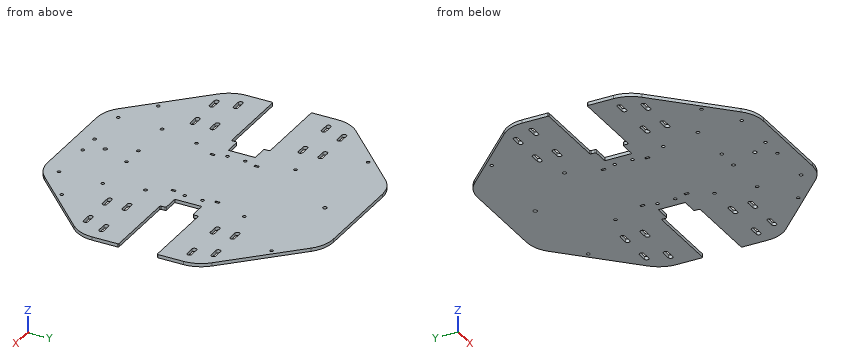
from build123d import *

# Parameters (mm, degrees)
SKETCH1_R           = 1.85
SKETCH1_R_2         = 1.5
BOSS_EXTRUDE1_DEPTH = 3
SKETCH2_R           = 1.5
SKETCH2_W           = 2
SKETCH2_H           = 4
CUT_EXTRUDE1_DEPTH  = 10
FILLET1_R           = 1
FILLET2_R           = 1
SKETCH3_R           = 1.5
CUT_EXTRUDE2_DEPTH  = 10


with BuildPart() as part:
    # Sketch1 → Boss-Extrude1 (new body)
    with BuildSketch(Plane.XY):
        with BuildLine():
            Line((130, 17.5), (130, 41.421356237))
            ThreePointArc((130, 41.421356237), (127.716385975, 52.901859208), (121.213203436, 62.634559673))
            Line((121.213203436, 62.634559673), (62.634559673, 121.213203436))
            ThreePointArc((62.634559673, 121.213203436), (52.901859208, 127.716385975), (41.421356237, 130))
            Line((41.421356237, 130), (-41.421356237, 130))
            ThreePointArc((-41.421356237, 130), (-52.901859208, 127.716385975), (-62.634559673, 121.213203436))
            Line((-62.634559673, 121.213203436), (-121.213203436, 62.634559673))
            ThreePointArc((-121.213203436, 62.634559673), (-127.716385975, 52.901859208), (-130, 41.421356237))
            Line((-130, 41.421356237), (-130, 17.5))
            Line((-130, 17.5), (-60, 17.5))
            Line((-60, 17.5), (-60, 12.25))
            Line((-60, 12.25), (-45, 12.25))
            Line((-45, 12.25), (-45, -12.25))
            Line((-45, -12.25), (-60, -12.25))
            Line((-60, -12.25), (-60, -17.5))
            Line((-60, -17.5), (-130, -17.5))
            Line((-130, -17.5), (-130, -41.421356237))
            ThreePointArc((-130, -41.421356237), (-127.716385975, -52.901859208), (-121.213203436, -62.634559673))
            Line((-121.213203436, -62.634559673), (-62.634559673, -121.213203436))
            ThreePointArc((-62.634559673, -121.213203436), (-52.901859208, -127.716385975), (-41.421356237, -130))
            Line((-41.421356237, -130), (41.421356237, -130))
            ThreePointArc((41.421356237, -130), (52.901859208, -127.716385975), (62.634559673, -121.213203436))
            Line((62.634559673, -121.213203436), (121.213203436, -62.634559673))
            ThreePointArc((121.213203436, -62.634559673), (127.716385975, -52.901859208), (130, -41.421356237))
            Line((130, -41.421356237), (130, -17.5))
            Line((130, -17.5), (60, -17.5))
            Line((60, -17.5), (60, -12.25))
            Line((60, -12.25), (45, -12.25))
            Line((45, -12.25), (45, 12.25))
            Line((45, 12.25), (60, 12.25))
            Line((60, 12.25), (60, 17.5))
            Line((60, 17.5), (130, 17.5))
        make_face()
        with Locations((0, 100)):
            Circle(SKETCH1_R, mode=Mode.SUBTRACT)
        with Locations(Location((0, -100, 0), (0, 0, 180))):
            Circle(SKETCH1_R, mode=Mode.SUBTRACT)
        with Locations((36, 8.1)):
            Circle(SKETCH1_R_2, mode=Mode.SUBTRACT)
        with Locations(Location((36, -8.1, 0), (0, 0, 180))):
            Circle(SKETCH1_R_2, mode=Mode.SUBTRACT)
        with Locations((-36, -8.1)):
            Circle(SKETCH1_R_2, mode=Mode.SUBTRACT)
        with Locations(Location((-36, 8.1, 0), (0, 0, 180))):
            Circle(SKETCH1_R_2, mode=Mode.SUBTRACT)
        with BuildLine():
            Line((69.925, 42.0875), (78.075, 42.0875))
            ThreePointArc((78.075, 42.0875), (80.1125, 40.05), (78.075, 38.0125))
            Line((78.075, 38.0125), (69.925, 38.0125))
            ThreePointArc((69.925, 38.0125), (67.8875, 40.05), (69.925, 42.0875))
        make_face(mode=Mode.SUBTRACT)
        with BuildLine():
            Line((69.925, 60.1375), (78.075, 60.1375))
            ThreePointArc((78.075, 60.1375), (80.1125, 58.1), (78.075, 56.0625))
            Line((78.075, 56.0625), (69.925, 56.0625))
            ThreePointArc((69.925, 56.0625), (67.8875, 58.1), (69.925, 60.1375))
        make_face(mode=Mode.SUBTRACT)
        with BuildLine():
            Line((101.925, 60.1375), (110.075, 60.1375))
            ThreePointArc((110.075, 60.1375), (112.1125, 58.1), (110.075, 56.0625))
            Line((110.075, 56.0625), (101.925, 56.0625))
            ThreePointArc((101.925, 56.0625), (99.8875, 58.1), (101.925, 60.1375))
        make_face(mode=Mode.SUBTRACT)
        with BuildLine():
            Line((108.925, 42.0875), (117.075, 42.0875))
            ThreePointArc((117.075, 42.0875), (119.1125, 40.05), (117.075, 38.0125))
            Line((117.075, 38.0125), (108.925, 38.0125))
            ThreePointArc((108.925, 38.0125), (106.8875, 40.05), (108.925, 42.0875))
        make_face(mode=Mode.SUBTRACT)
        with BuildLine():
            Line((-69.925, 60.1375), (-78.075, 60.1375))
            ThreePointArc((-78.075, 60.1375), (-80.1125, 58.1), (-78.075, 56.0625))
            Line((-78.075, 56.0625), (-69.925, 56.0625))
            ThreePointArc((-69.925, 56.0625), (-67.8875, 58.1), (-69.925, 60.1375))
        make_face(mode=Mode.SUBTRACT)
        with BuildLine():
            Line((-101.925, 60.1375), (-110.075, 60.1375))
            ThreePointArc((-110.075, 60.1375), (-112.1125, 58.1), (-110.075, 56.0625))
            Line((-110.075, 56.0625), (-101.925, 56.0625))
            ThreePointArc((-101.925, 56.0625), (-99.8875, 58.1), (-101.925, 60.1375))
        make_face(mode=Mode.SUBTRACT)
        with BuildLine():
            Line((-108.925, 42.0875), (-117.075, 42.0875))
            ThreePointArc((-117.075, 42.0875), (-119.1125, 40.05), (-117.075, 38.0125))
            Line((-117.075, 38.0125), (-108.925, 38.0125))
            ThreePointArc((-108.925, 38.0125), (-106.8875, 40.05), (-108.925, 42.0875))
        make_face(mode=Mode.SUBTRACT)
        with BuildLine():
            Line((-69.925, 42.0875), (-78.075, 42.0875))
            ThreePointArc((-78.075, 42.0875), (-80.1125, 40.05), (-78.075, 38.0125))
            Line((-78.075, 38.0125), (-69.925, 38.0125))
            ThreePointArc((-69.925, 38.0125), (-67.8875, 40.05), (-69.925, 42.0875))
        make_face(mode=Mode.SUBTRACT)
        with BuildLine():
            Line((101.925, -60.1375), (110.075, -60.1375))
            ThreePointArc((110.075, -60.1375), (112.1125, -58.1), (110.075, -56.0625))
            Line((110.075, -56.0625), (101.925, -56.0625))
            ThreePointArc((101.925, -56.0625), (99.8875, -58.1), (101.925, -60.1375))
        make_face(mode=Mode.SUBTRACT)
        with BuildLine():
            Line((69.925, -60.1375), (78.075, -60.1375))
            ThreePointArc((78.075, -60.1375), (80.1125, -58.1), (78.075, -56.0625))
            Line((78.075, -56.0625), (69.925, -56.0625))
            ThreePointArc((69.925, -56.0625), (67.8875, -58.1), (69.925, -60.1375))
        make_face(mode=Mode.SUBTRACT)
        with BuildLine():
            Line((69.925, -42.0875), (78.075, -42.0875))
            ThreePointArc((78.075, -42.0875), (80.1125, -40.05), (78.075, -38.0125))
            Line((78.075, -38.0125), (69.925, -38.0125))
            ThreePointArc((69.925, -38.0125), (67.8875, -40.05), (69.925, -42.0875))
        make_face(mode=Mode.SUBTRACT)
        with BuildLine():
            Line((108.925, -42.0875), (117.075, -42.0875))
            ThreePointArc((117.075, -42.0875), (119.1125, -40.05), (117.075, -38.0125))
            Line((117.075, -38.0125), (108.925, -38.0125))
            ThreePointArc((108.925, -38.0125), (106.8875, -40.05), (108.925, -42.0875))
        make_face(mode=Mode.SUBTRACT)
        with BuildLine():
            Line((-101.925, -60.1375), (-110.075, -60.1375))
            ThreePointArc((-110.075, -60.1375), (-112.1125, -58.1), (-110.075, -56.0625))
            Line((-110.075, -56.0625), (-101.925, -56.0625))
            ThreePointArc((-101.925, -56.0625), (-99.8875, -58.1), (-101.925, -60.1375))
        make_face(mode=Mode.SUBTRACT)
        with BuildLine():
            Line((-69.925, -60.1375), (-78.075, -60.1375))
            ThreePointArc((-78.075, -60.1375), (-80.1125, -58.1), (-78.075, -56.0625))
            Line((-78.075, -56.0625), (-69.925, -56.0625))
            ThreePointArc((-69.925, -56.0625), (-67.8875, -58.1), (-69.925, -60.1375))
        make_face(mode=Mode.SUBTRACT)
        with BuildLine():
            Line((-69.925, -42.0875), (-78.075, -42.0875))
            ThreePointArc((-78.075, -42.0875), (-80.1125, -40.05), (-78.075, -38.0125))
            Line((-78.075, -38.0125), (-69.925, -38.0125))
            ThreePointArc((-69.925, -38.0125), (-67.8875, -40.05), (-69.925, -42.0875))
        make_face(mode=Mode.SUBTRACT)
        with BuildLine():
            Line((-108.925, -42.0875), (-117.075, -42.0875))
            ThreePointArc((-117.075, -42.0875), (-119.1125, -40.05), (-117.075, -38.0125))
            Line((-117.075, -38.0125), (-108.925, -38.0125))
            ThreePointArc((-108.925, -38.0125), (-106.8875, -40.05), (-108.925, -42.0875))
        make_face(mode=Mode.SUBTRACT)
    extrude(amount=BOSS_EXTRUDE1_DEPTH)

    # Sketch2 → Cut-Extrude1 (cut)
    with BuildSketch(Plane.XY.offset(3)):
        with Locations((-10, -75.1)):
            Circle(SKETCH2_R)
        with Locations((-49.9, -75.1)):
            Circle(SKETCH2_R)
        with Locations((-10, -115)):
            Circle(SKETCH2_R)
        with Locations((-49.9, -115)):
            Circle(SKETCH2_R)
        with Locations((10, -75.1)):
            Circle(SKETCH2_R)
        with Locations((49.9, -75.1)):
            Circle(SKETCH2_R)
        with Locations((49.9, -115)):
            Circle(SKETCH2_R)
        with Locations((10, -115)):
            Circle(SKETCH2_R)
        with Locations((33, -20)):
            Rectangle(SKETCH2_W, SKETCH2_H)
        with Locations((33, 20)):
            Rectangle(SKETCH2_W, SKETCH2_H)
        with Locations((-33, 20)):
            Rectangle(SKETCH2_W, SKETCH2_H)
        with Locations((-33, -20)):
            Rectangle(SKETCH2_W, SKETCH2_H)
    extrude(amount=-CUT_EXTRUDE1_DEPTH, mode=Mode.SUBTRACT)

    # Fillet1
    fillet1_edges = [part.edges().sort_by_distance(p)[0] for p in [
        (130, 17.5, 1.5),
        (60, 17.5, 1.5),
        (60, 12.25, 1.5),
        (60, -12.25, 1.5),
        (60, -17.5, 1.5),
        (130, -17.5, 1.5),
    ]]
    fillet(fillet1_edges, radius=FILLET1_R)

    # Fillet2
    fillet2_edges = [part.edges().sort_by_distance(p)[0] for p in [
        (-130, -17.5, 1.5),
        (-60, -17.5, 1.5),
        (-60, -12.25, 1.5),
        (-60, 12.25, 1.5),
        (-60, 17.5, 1.5),
        (-130, 17.5, 1.5),
    ]]
    fillet(fillet2_edges, radius=FILLET2_R)

    # Sketch3 → Cut-Extrude2 (cut)
    with BuildSketch(Plane.XY.offset(3)):
        with Locations((-43, 50)):
            Circle(SKETCH3_R)
        with Locations((-43, -40)):
            Circle(SKETCH3_R)
        with Locations((43, -40)):
            Circle(SKETCH3_R)
        with Locations((43, 50)):
            Circle(SKETCH3_R)
        with Locations((-81.317279836, 95.45941546)):
            Circle(SKETCH3_R)
        with Locations((81.317279836, 95.45941546)):
            Circle(SKETCH3_R)
        with Locations((81.317279836, -95.45941546)):
            Circle(SKETCH3_R)
        with Locations((-81.317279836, -95.45941546)):
            Circle(SKETCH3_R)
    extrude(amount=-CUT_EXTRUDE2_DEPTH, mode=Mode.SUBTRACT)


solid = part.part
Can you work these out from the model? Positions are in its coordinate system, mm. Give positions to 0.01 mm unless a question says otherwise; leave off trailing zeros. Loops run counter-clockwise (first coordinate to the right, second up) from the corner with the lowest first, then second, coordinate; pieces in that order, holes last. Notation, with made-up numbers: (26, -14.5) - (44, -14.5) arc R24 ccw to (44, -4.5) - close; hole circle Ø3 at (61, 1.5). An arc over 180 degrees is marked (long way). Answer as a JSON object with one key per item and string values.
Q1. Will these pins go through, and if not, where does the flat tip stop? P1, Ø0.9, axis at x = 108, z = 2, coming from the -Y side; P2, Ø1, axis at x = -46.5, z = 2.5, coming from the +Y side; P3, Ø1.5, axis at x = 105, z = 1.5, coming from the +Y side.
Geometry says:
{"P1": "y = -76.3", "P2": "y = 129.65", "P3": "y = 79.6"}
Q2. Imagine slicing it at C-C on y = 77.5. Write out the boundary of the cut face in (x, z), plus the area to 3 significant figures.
Geometry says:
{"outline": "(-106.35, 0) - (106.35, 0) - (106.35, 3) - (-106.35, 3) - close", "area": "638 mm²"}
Q3. If I drill on L1, parallel to X at y = -21, z = 2.6; L2, parallel to Y at x = 10, z = 1.3; L3, parallel to Y at x = 36, z = 0.7, over which ranges is the centre line in solid material (lowest first)?
Geometry says:
{"L1": "-130 to -34, -32 to 32, 34 to 130", "L2": "-130 to -116.5, -113.5 to -76.6, -73.6 to 130", "L3": "-130 to -9.6, -6.6 to 6.6, 9.6 to 130"}
Q4. Imagine slicing it at A-A on z = 1. Give the number of separate pieces and of enclosed holes in the cut face, plus the area to 3 significant figures.
Geometry says:
{"separate pieces": "1", "enclosed holes": "42", "area": "49,300 mm²"}
Q5. Imagine slicing it at B-B on y = -108.5. Write out the boundary of the cut face in (x, z), plus the area to 3 significant figures.
Geometry says:
{"outline": "(-75.35, 0) - (75.35, 0) - (75.35, 3) - (-75.35, 3) - close", "area": "452 mm²"}
